Model file for the job. Use its own axes, mm. A direction names the side the tool comes from. Coordinates: 2 decimals unless noted, no trailing zeros. Write each loop counter-clockwise with the first axis right and the second up, starting at its lowest first coordinate (ties: lowest second). Pieces come first, ordered by that corner, then holes. Notation, with made-up numbers: (-10, -20) -> (4, -20) arc R29 ccw to (4, 15) -> close; hole circle Ø10 at (71.5, -28). An arc over 180 degrees is marked (long way). Answer as a JSON object with one key per item and string values. Group by question number.
from build123d import *

# Parameters (mm, degrees)
SKETCH1_R           = 17.5
BOSS_EXTRUDE1_DEPTH = 20
BOSS_EXTRUDE2_START = 8.5
SKETCH2_R           = 17.5
BOSS_EXTRUDE2_DEPTH = 8.5
BOSS_EXTRUDE3_DEPTH = 12
SKETCH4_R           = 3
CUT_EXTRUDE1_DEPTH  = 186.350058538
SKETCH5_R           = 1.75
CUT_EXTRUDE2_DEPTH  = 186.288354194
FILLET1_R           = 10


with BuildPart() as part:
    # Sketch1 → Boss-Extrude1 (new body)
    with BuildSketch(Plane(origin=(0, 0, 0), x_dir=(1, 0, 0), z_dir=(0, 1, 0))):
        Circle(SKETCH1_R)
        with BuildLine():
            Line((67.5, 17.5), (0, 17.5))
            ThreePointArc((0, 17.5), (12.374368671, 12.374368671), (17.5, 0))
            ThreePointArc((17.5, 0), (12.374368671, -12.374368671), (0, -17.5))
            Line((0, -17.5), (67.5, -17.5))
            Line((67.5, -17.5), (67.5, 17.5))
        make_face()
    extrude(amount=BOSS_EXTRUDE1_DEPTH)

    # Sketch2 → Boss-Extrude2 (add)
    with BuildSketch(Plane.XZ.offset(BOSS_EXTRUDE2_START)):
        with Locations(Location((0, 0, 0), (0, 0, 270))):
            Circle(SKETCH2_R)
    extrude(amount=-BOSS_EXTRUDE2_DEPTH)

    # Sketch3 → Boss-Extrude3 (add)
    with BuildSketch(Plane(origin=(67.5, 0, 0), x_dir=(0, 0, -1), z_dir=(1, 0, 0))):
        Polygon((17.5, 0), (17.5, 20), (17.5, 114.118307847), (-12.79, 151.39), (-64.89, 151.39), (-64.89, 76.846615693), (-57.39, 67.85), (-17.5, 20), (-17.5, 0), align=None)
    extrude(amount=-BOSS_EXTRUDE3_DEPTH)

    # Sketch4 → Cut-Extrude1 (cut, through all)
    with BuildSketch(Plane(origin=(67.5, 0, 0), x_dir=(0, 0, -1), z_dir=(1, 0, 0))):
        with Locations((-56.89, 101.418307847)):
            Circle(SKETCH4_R)
        with Locations((-56.89, 126.818307847)):
            Circle(SKETCH4_R)
        with Locations((-31.49, 114.118307847)):
            Circle(SKETCH4_R)
    extrude(amount=-CUT_EXTRUDE1_DEPTH, mode=Mode.SUBTRACT)

    # Sketch5 → Cut-Extrude2 (cut, through all)
    with BuildSketch(Plane.XZ.offset(8.5)):
        with Locations(Location((0, 12.5, 0), (0, 0, 270))):
            Circle(SKETCH5_R)
        with Locations(Location((10.825317547, 6.25, 0), (0, 0, 270))):
            Circle(SKETCH5_R)
        with Locations(Location((10.825317547, -6.25, 0), (0, 0, 270))):
            Circle(SKETCH5_R)
        with Locations(Location((0, -12.5, 0), (0, 0, 270))):
            Circle(SKETCH5_R)
        with Locations(Location((-10.825317547, -6.25, 0), (0, 0, 270))):
            Circle(SKETCH5_R)
        with Locations(Location((-10.825317547, 6.25, 0), (0, 0, 270))):
            Circle(SKETCH5_R)
    extrude(amount=-CUT_EXTRUDE2_DEPTH, mode=Mode.SUBTRACT)

    # Fillet1
    # the kernel refuses this fillet: 10 mm, written as the material it adds along each edge
    with BuildSketch(Plane(origin=(55.5, 20, 42.5), x_dir=(-1, 0, 0), z_dir=(0, 0, -1))) as fillet1_piece_1_section:
        with BuildLine():
            CenterArc((FILLET1_R, FILLET1_R), FILLET1_R, 180, 90)
            Line((0, FILLET1_R), (0, 0))
            Line((0, 0), (FILLET1_R, 0))
        make_face()
    fillet1_piece_1 = extrude(amount=60, mode=Mode.PRIVATE)
    fillet1_piece_1 = split(fillet1_piece_1, bisect_by=Plane(origin=(54.435274847, 24.301180518, 17.5), z_dir=(0, 0, 1)), keep=Keep.TOP, mode=Mode.PRIVATE)
    fillet1_piece_1 = split(fillet1_piece_1, bisect_by=Plane(origin=(54.435274847, 23.419399768, 20.350571719), z_dir=(0, 0.6403264910942221, -0.7681028478029236)), keep=Keep.TOP, mode=Mode.PRIVATE)
    add(fillet1_piece_1)
    with BuildSketch(Plane(origin=(55.5, 20, 17.5), x_dir=(-1, 0, 0), z_dir=(0, 0, -1))) as fillet1_piece_2_section:
        with BuildLine():
            CenterArc((FILLET1_R, FILLET1_R), FILLET1_R, 180, 90)
            Line((0, FILLET1_R), (0, 0))
            Line((0, 0), (FILLET1_R, 0))
        make_face()
    fillet1_piece_2 = extrude(amount=35, mode=Mode.PRIVATE)
    fillet1_piece_2 = split(fillet1_piece_2, bisect_by=Plane(origin=(53.236551243, 12.727184254, 11.437040332), z_dir=(0, 0.6403264910942221, -0.7681028478029236)), keep=Keep.TOP, mode=Mode.PRIVATE)
    add(fillet1_piece_2)


with BuildPart() as body_2:
    # Mirror1: mirrored copy
    add(part.part.mirror(Plane(origin=(-20, 0, 0), x_dir=(0, 0, 1), z_dir=(1, 0, 0))))


solid = body_2.part
(1) 3-axis set-ups, long thin cutter, end or side, ignore diameter. For faces 4 (the face through (-24.474, 2.384, -8.075)), 5 (the face through (-54, 20, 0)), 6 (the face through (-73, 10, 17.5)): which of +Z, -Z, +X, -X, +Y, -Y reach the whole face in a straight line?
(2) Wall check: probe 1 along Z at (x, y) = (-40, 10.75); probe 2 along X at (y, z) = (80, -9); probe 3 along Y at (x, z) = (-100.5, 56.5). Give the ranges that are in metal, low to high.
(3) Cut at B-B on z = 6.25. List the corners of the cut face in (x, y), plus the area to 3 significant figures.
(4) Cut at A-A on z = 32.5. List the corners of the cut face in (x, y).
(5) Pull direction X, two halves, no side cores. Call faces 1 (the face through (-50.9, 5.6, -4.5)), 2 (the face through (-102, 115, 64.89)), 3 (the face through (-92.65, 23.01, -0.34)): released by +X, released by -X, zero draft, split by the parting line, or undercut.
(6) Cut at D-D on x = -75. List the corners of the cut face in (y, z).
(7) Pin check, flat tips, straight feed: pin 1 (17.5 mm diameter, centred on x = -48.5, z = 5, fed in from +Y); pin 2 (5 mm diameter, centred on x = -84, z = 13, fed in from -Y); pin 3 (4 mm diameter, centred on y = 61, z = 23.5, fed in from +X). Stop position of each tip, or through.
(8) Cut at C-C on y = 90.5. List the corners of the cut face in (x, z), plus the area to 3 significant figures.
Results found:
{
 "1": {"face 4": "-Y", "face 5": "+Z, -Z, +X, +Y", "face 6": "+Z, +X, -X, -Y"},
 "2": {"probe 1": "z = -17.5 to -14.25, -10.75 to 10.75, 14.25 to 17.5", "probe 2": "x = -107.5 to -95.5", "probe 3": "y = 66.78 to 98.44, 104.39 to 123.84, 129.79 to 151.39"},
 "3": {"outline": "(-107.5, 0) -> (-56.35, 0) -> (-56.35, -8.5) -> (-52.58, -8.5) -> (-52.58, 20) -> (-85.5, 20) arc R10 cw to (-95.5, 30) -> (-95.5, 143.34) -> (-107.5, 143.34) -> close; (-49.08, -8.5) -> (-30.92, -8.5) -> (-30.92, 20) -> (-49.08, 20) -> close; (-27.42, -8.5) -> (-23.65, -8.5) -> (-23.65, 20) -> (-27.42, 20) -> close", "area": "3,260 mm²"},
 "4": {"outline": "(-107.5, 37.99) -> (-95.5, 37.99) -> (-95.5, 111.29) -> (-107.5, 111.29) -> close; (-107.5, 116.94) -> (-95.5, 116.94) -> (-95.5, 151.39) -> (-107.5, 151.39) -> close"},
 "5": {"face 1": "undercut", "face 2": "zero draft", "face 3": "released by +X"},
 "6": {"outline": "(0, -17.5) -> (20, -17.5) -> (20, 17.5) -> (0, 17.5) -> close"},
 "7": {"pin 1": "stops at y = 20", "pin 2": "stops at y = 0", "pin 3": "stops at x = -95.5"},
 "8": {"outline": "(-107.5, -17.5) -> (-95.5, -17.5) -> (-95.5, 64.89) -> (-107.5, 64.89) -> close", "area": "989 mm²"}
}
